For this review, take the finished solid that the model builds, in its own axes (mm). Give positions to 0.01 mm unless a question says otherwise; leave off trailing zeros. Order: outer loops, then holes, each group sorted by start corner. A loop starts at its lowest first (then second) coordinate and runs counter-clockwise, first axis right, second up.
Item 1: Consider section A-A (y = 140). Give the boundary of the cut face in (x, z), plus the area to 3 significant figures.
Item 2: For P1, Ø1.2, axis at y = 231.5, z = 2, coming from the +X side; P2, Ø1, axis at x = 23.5, z = 2.5, coming from the -Y side; P3, Ø2, axis at x = -15.5, z = 2.5, coming from the +Y side, all flat-tipped, find the tip position at first contact; note any pin that passes through.
Item 3: Consider section B-B (y = 178). Give the boundary of the cut face in (x, z), plus the area to 3 significant figures.
Item 4: For probe 1 along X at (y, z) = (166, 1.6); probe 2 along X at (y, z) = (231, 1.3); probe 3 along X at (y, z) = (221, 0.85), list the stretches that pass through material, from the lowest coordinate up.
Item 5: Consider section C-C (z = 1.15). Give the number of separate pieces and of enclosed holes in the cut face, plus the area to 3 significant figures.
```python
from build123d import *

# Parameters (mm, degrees)
SKETCH1_R           = 4
SKETCH1_R_2         = 11
SKETCH1_R_3         = 1.5
SKETCH1_W           = 4
SKETCH1_H           = 30
SKETCH1_W_2         = 8.515362535
SKETCH1_H_2         = 50.591793773
SKETCH1_W_3         = 9.363802293
SKETCH1_H_3         = 53.507441676
SKETCH1_H_4         = 49.971994441
BOSS_EXTRUDE1_DEPTH = 4


with BuildPart() as part:
    # Sketch1 → Boss-Extrude1 (new body)
    with BuildSketch(Plane.XY):
        with BuildLine():
            Line((-35, 300), (-35, 245.119310596))
            Line((-35, 245.119310596), (-31, 245.119310596))
            Line((-31, 245.119310596), (-31, 225.119310596))
            Line((-31, 225.119310596), (-35, 225.119310596))
            Line((-35, 225.119310596), (-35, 185.119310596))
            Line((-35, 185.119310596), (-31, 185.119310596))
            Line((-31, 185.119310596), (-31, 165.119310596))
            Line((-31, 165.119310596), (-35, 165.119310596))
            Line((-35, 165.119310596), (-35, 125.119310596))
            Line((-35, 125.119310596), (-31, 125.119310596))
            Line((-31, 125.119310596), (-31, 105.119310596))
            Line((-31, 105.119310596), (-35, 105.119310596))
            Line((-35, 105.119310596), (-35, 65.119310596))
            Line((-35, 65.119310596), (-31, 65.119310596))
            Line((-31, 65.119310596), (-31, 45.119310596))
            Line((-31, 45.119310596), (-35, 45.119310596))
            Line((-35, 45.119310596), (-35, 0))
            Line((-35, 0), (-23, 0))
            ThreePointArc((-23, 0), (-22.921443339, -1.899324946), (-22.686309978, -3.785675576))
            Line((-22.686309978, -3.785675576), (-34.522645619, -5.76081066))
            ThreePointArc((-34.522645619, -5.76081066), (-33.929009308, -8.59199205), (-33.10360346, -11.364481422))
            Line((-33.10360346, -11.364481422), (-21.753796559, -7.468087792))
            ThreePointArc((-21.753796559, -7.468087792), (-21.062786513, -9.238994767), (-20.227896278, -10.94679004))
            Line((-20.227896278, -10.94679004), (-30.781581292, -16.658158756))
            ThreePointArc((-30.781581292, -16.658158756), (-29.300826739, -19.143185534), (-27.619917829, -21.497444944))
            Line((-27.619917829, -21.497444944), (-18.150231716, -14.126892392))
            ThreePointArc((-18.150231716, -14.126892392), (-16.921649945, -15.577476147), (-15.577476147, -16.921649945))
            Line((-15.577476147, -16.921649945), (-23.704855007, -25.750336874))
            ThreePointArc((-23.704855007, -25.750336874), (-21.497444944, -27.619917829), (-19.143185534, -29.300826739))
            Line((-19.143185534, -29.300826739), (-12.579807637, -19.254829))
            ThreePointArc((-12.579807637, -19.254829), (-10.94679004, -20.227896278), (-9.238994767, -21.062786513))
            Line((-9.238994767, -21.062786513), (-14.059339863, -32.052066433))
            ThreePointArc((-14.059339863, -32.052066433), (-11.364481422, -33.10360346), (-8.59199205, -33.929009308))
            Line((-8.59199205, -33.929009308), (-5.646166204, -22.296206117))
            ThreePointArc((-5.646166204, -22.296206117), (-3.785675576, -22.686309978), (-1.899324946, -22.921443339))
            Line((-1.899324946, -22.921443339), (-2.890277092, -34.880457255))
            ThreePointArc((-2.890277092, -34.880457255), (0, -35), (2.890277092, -34.880457255))
            Line((2.890277092, -34.880457255), (1.899324946, -22.921443339))
            ThreePointArc((1.899324946, -22.921443339), (3.785675576, -22.686309978), (5.646166204, -22.296206117))
            Line((5.646166204, -22.296206117), (8.59199205, -33.929009308))
            ThreePointArc((8.59199205, -33.929009308), (11.364481422, -33.10360346), (14.059339863, -32.052066433))
            Line((14.059339863, -32.052066433), (9.238994767, -21.062786513))
            ThreePointArc((9.238994767, -21.062786513), (10.94679004, -20.227896278), (12.579807637, -19.254829))
            Line((12.579807637, -19.254829), (19.143185534, -29.300826739))
            ThreePointArc((19.143185534, -29.300826739), (21.497444944, -27.619917829), (23.704855007, -25.750336874))
            Line((23.704855007, -25.750336874), (15.577476147, -16.921649945))
            ThreePointArc((15.577476147, -16.921649945), (16.921649945, -15.577476147), (18.150231716, -14.126892392))
            Line((18.150231716, -14.126892392), (27.619917829, -21.497444944))
            ThreePointArc((27.619917829, -21.497444944), (29.300826739, -19.143185534), (30.781581292, -16.658158756))
            Line((30.781581292, -16.658158756), (20.227896278, -10.94679004))
            ThreePointArc((20.227896278, -10.94679004), (21.062786513, -9.238994767), (21.753796559, -7.468087792))
            Line((21.753796559, -7.468087792), (33.10360346, -11.364481422))
            ThreePointArc((33.10360346, -11.364481422), (33.929009308, -8.59199205), (34.522645619, -5.76081066))
            Line((34.522645619, -5.76081066), (22.686309978, -3.785675576))
            ThreePointArc((22.686309978, -3.785675576), (22.921443339, -1.899324946), (23, 0))
            Line((23, 0), (35, 0))
            Line((35, 0), (35, 45.119310596))
            Line((35, 45.119310596), (31, 45.119310596))
            Line((31, 45.119310596), (31, 65.119310596))
            Line((31, 65.119310596), (35, 65.119310596))
            Line((35, 65.119310596), (35, 105.119310596))
            Line((35, 105.119310596), (31, 105.119310596))
            Line((31, 105.119310596), (31, 125.119310596))
            Line((31, 125.119310596), (35, 125.119310596))
            Line((35, 125.119310596), (35, 165.119310596))
            Line((35, 165.119310596), (31, 165.119310596))
            Line((31, 165.119310596), (31, 185.119310596))
            Line((31, 185.119310596), (35, 185.119310596))
            Line((35, 185.119310596), (35, 225.119310596))
            Line((35, 225.119310596), (31, 225.119310596))
            Line((31, 225.119310596), (31, 245.119310596))
            Line((31, 245.119310596), (35, 245.119310596))
            Line((35, 245.119310596), (35, 300))
            ThreePointArc((35, 300), (0, 335), (-35, 300))
        make_face()
        Circle(SKETCH1_R, mode=Mode.SUBTRACT)
        with Locations((0, 300)):
            Circle(SKETCH1_R_2, mode=Mode.SUBTRACT)
        with Locations((23.996702537, 235.091311609)):
            Circle(SKETCH1_R_3, mode=Mode.SUBTRACT)
        with Locations((-24.57592592, 165.712200906)):
            Circle(SKETCH1_R_3, mode=Mode.SUBTRACT)
        with Locations((23.996702545, 199.384614522)):
            Circle(SKETCH1_R_3, mode=Mode.SUBTRACT)
        with Locations((-24.57592592, 130.741920595)):
            Circle(SKETCH1_R_3, mode=Mode.SUBTRACT)
        with Locations((23.996702545, 70.517408204)):
            Circle(SKETCH1_R_3, mode=Mode.SUBTRACT)
        with Locations((23.834109516, 30.143932105)):
            Circle(SKETCH1_R_3, mode=Mode.SUBTRACT)
        with Locations((0, 236.5)):
            Rectangle(SKETCH1_W, SKETCH1_H, mode=Mode.SUBTRACT)
        with Locations((-15.100973899, 244.828514205)):
            Rectangle(SKETCH1_W_2, SKETCH1_H_2, mode=Mode.SUBTRACT)
        with Locations((11.541273102, 143.451426266)):
            Rectangle(SKETCH1_W_3, SKETCH1_H_3, mode=Mode.SUBTRACT)
        with Locations((-15.100973899, 60.133313376)):
            Rectangle(SKETCH1_W_2, SKETCH1_H_4, mode=Mode.SUBTRACT)
    extrude(amount=BOSS_EXTRUDE1_DEPTH)


solid = part.part
```
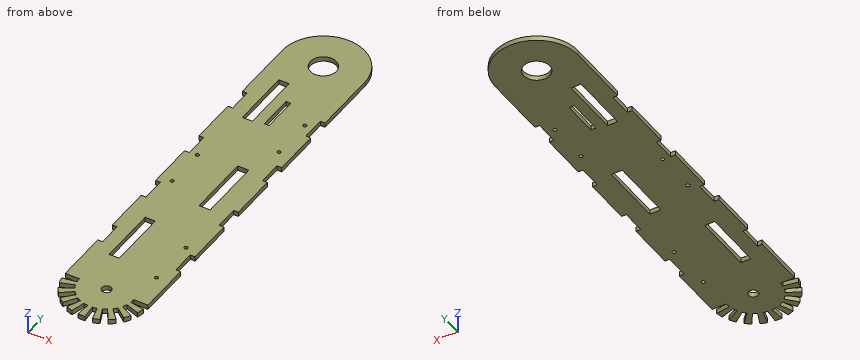
Resolved:
1. outline: (-35, 0) - (6.86, 0) - (6.86, 4) - (-35, 4) - close; (16.22, 0) - (35, 0) - (35, 4) - (16.22, 4) - close
1. area: 243 mm2
2. P1: stops at x = 31
2. P2: stops at y = -26.38
2. P3: stops at y = 331.86
3. outline: (-31, 0) - (31, 0) - (31, 4) - (-31, 4) - close
3. area: 248 mm2
4. probe 1: x = -31 to -26.05, -23.1 to 6.86, 16.22 to 31
4. probe 2: x = -31 to -19.36, -10.84 to -2, 2 to 31
4. probe 3: x = -35 to -19.36, -10.84 to 35
5. separate pieces: 1
5. enclosed holes: 12
5. area: 21,700 mm2
